Verification items for the finished model (mm, model axes). Face numbers are marked on the shaded views. A direction names the side the tool comes from. Round coordinates to 2 decimals unless told otherwise and drop trailing zeros. Loops run counter-clockwise (first coordinate to the right, second up) from the corner with the lowest first, then second, coordinate; pieces in that order, holes last. Notation, with made-up numbers: (29, 10.5) -> (77, 10.5) arc R8 ccw to (77, 22.5) -> close; hole circle Ø2 at (9.5, 43.5). An arc over 180 degrees is marked (long way). Write item = value, one per line.
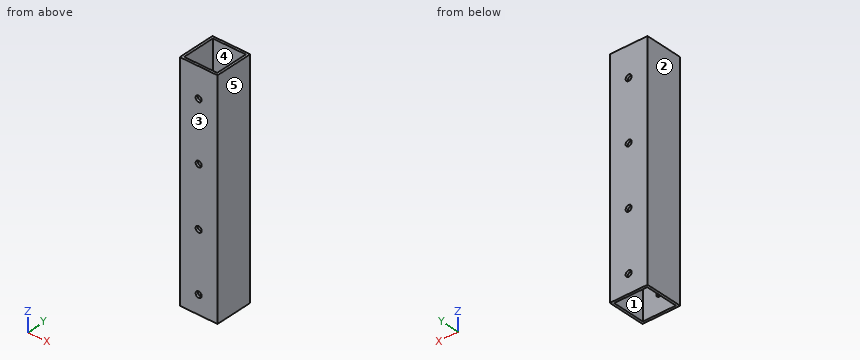
```python
from build123d import *

# Parameters (mm, degrees)
SKETCH1_W               = 50.8
SKETCH1_H               = 50.8
SKETCH1_W_2             = 44.45
SKETCH1_H_2             = 44.45
BOSS_EXTRUDE1_DEPTH     = 304.8
CUT_EXTRUDE1_DEPTH      = 304.8
CUT_EXTRUDE1_DEPTH_BACK = 304.8
SKETCH2_R               = 4.05


with BuildPart() as part:
    # Sketch1 → Boss-Extrude1 (new body)
    with BuildSketch(Plane.XY):
        Rectangle(SKETCH1_W, SKETCH1_H)
        Rectangle(SKETCH1_W_2, SKETCH1_H_2, mode=Mode.SUBTRACT)
    extrude(amount=-BOSS_EXTRUDE1_DEPTH)

    # Sketch2 → Cut-Extrude1 (cut, two sides: drawn at the far end of the back side and taken through both)
    with BuildSketch(Plane(origin=(0, 0, 0), x_dir=(1, 0, 0), z_dir=(0, 1, 0)).offset(-CUT_EXTRUDE1_DEPTH_BACK)):
        with Locations(Location((0, 40, 0), (0, 0, 90))):
            Circle(SKETCH2_R)
        with Locations(Location((0, 120, 0), (0, 0, 90))):
            Circle(SKETCH2_R)
        with Locations(Location((0, 200, 0), (0, 0, 90))):
            Circle(SKETCH2_R)
        with Locations(Location((0, 280, 0), (0, 0, 90))):
            Circle(SKETCH2_R)
    extrude(amount=CUT_EXTRUDE1_DEPTH + CUT_EXTRUDE1_DEPTH_BACK, mode=Mode.SUBTRACT)


solid = part.part
```
(1) Set-up check for the marked faces 4 and 5: record each of +Z, -Z, +X, -X, +Y, -Y from which the full face is reachable in a straight line by a thin tool's end or side.
Filled sheet:
face_4 = +Z, -Z
face_5 = +Z, -Z, +X, +Y, -Y
(2) Sectioned sample at A-A, the plane x = -19. Record the cut outline in (y, z) (3 decimals), and give its area (3 significant figures).
Filled sheet:
outline = (-25.4, -304.8) -> (-22.225, -304.8) -> (-22.225, 0) -> (-25.4, 0) -> close; (22.225, -304.8) -> (25.4, -304.8) -> (25.4, 0) -> (22.225, 0) -> close
area = 1,940 mm2
(3) Draft check along Y on the marked faces 1, 2 and 3. Enter one of: released by +Y, released by -Y, zero draft, split by the parting line, or undercut.
Filled sheet:
face_1 = undercut
face_2 = zero draft
face_3 = released by -Y
(4) Go/stop test with a flat-tipped pin: pin 1 Ø9.5 at (x, z) = (0, -120) entering from +Y. Record where the tip stops, or that it passes through.
Filled sheet:
pin_1 = 25.4
(5) Sectioned sample at B-B, the plane z = -78. Record the cut outline in (x, y) (3 decimals), and give its area (3 significant figures).
Filled sheet:
outline = (-25.4, -25.4) -> (25.4, -25.4) -> (25.4, 25.4) -> (-25.4, 25.4) -> close; hole (-22.225, -22.225) -> (22.225, -22.225) -> (22.225, 22.225) -> (-22.225, 22.225) -> close
area = 605 mm2
(6) Sectioned sample at D-D, the plane z = -200. Record the cut outline in (x, y) (3 decimals), and give its area (3 significant figures).
Filled sheet:
outline = (-25.4, -25.4) -> (-4.05, -25.4) -> (-4.05, -22.225) -> (-22.225, -22.225) -> (-22.225, 22.225) -> (-4.05, 22.225) -> (-4.05, 25.4) -> (-25.4, 25.4) -> close; (4.05, -25.4) -> (25.4, -25.4) -> (25.4, 25.4) -> (4.05, 25.4) -> (4.05, 22.225) -> (22.225, 22.225) -> (22.225, -22.225) -> (4.05, -22.225) -> close
area = 553 mm2
(7) Material ranges on probe 1 along X at (y, z) = (21.5, -180) (3 decimals); probe 2 along X at (y, z) = (23.25, -200), recorded low to high. Write a range as from..to.
Filled sheet:
probe_1 = -25.4..-22.225, 22.225..25.4
probe_2 = -25.4..-4.05, 4.05..25.4
